from build123d import *

# Parameters (mm, degrees)
F0_R     = 11
F0_R_2   = 8.85
F0_R_3   = 8.1
F0_R_4   = 5
F1_DEPTH = 1.5
F2_DEPTH = 2.65
F3_DEPTH = 1
F4_DEPTH = 0.8


with BuildPart() as f1:
    # F0 (on Top) → F1 (new body)
    with BuildSketch(Plane.XY):
        Circle(F0_R)
        Circle(F0_R_2, mode=Mode.SUBTRACT)
        Circle(F0_R_2)
        Circle(F0_R_3, mode=Mode.SUBTRACT)
        Circle(F0_R_3)
        Circle(F0_R_4, mode=Mode.SUBTRACT)
    extrude(amount=-F1_DEPTH)

    # F0 (on Top) → F2 (join)
    with BuildSketch(Plane.XY):
        Circle(F0_R_2)
        Circle(F0_R_3, mode=Mode.SUBTRACT)
    extrude(amount=F2_DEPTH)

    # F3 (add): a face of the model
    f3_faces = [f1.faces().sort_by_distance(p)[0] for p in [
        (-8.5996841995, 0, 2.65),
    ]]
    extrude(f3_faces, amount=F3_DEPTH)

    # F4 (add): a face of the model
    f4_faces = [f1.faces().sort_by_distance(p)[0] for p in [
        (-7.8708974029, 0, 0),
    ]]
    extrude(f4_faces, amount=F4_DEPTH)


solid = f1.part
The listing builds one solid part. Answer for the finished solid, in the listing's coordinates (mm). A direction names the side the tool comes from. Round coordinates to 2 decimals unless told otherwise and drop trailing zeros. Write each loop counter-clockwise with the first axis right and the second up, starting at its lowest first coordinate (ties: lowest second). Pieces come first, ordered by that corner, then holes. Notation, with made-up numbers: (31.5, 53) - (76.5, 53) arc R32 cw to (76.5, 79) - close; hole circle Ø2 at (61.25, 68.25). An arc over 180 degrees is marked (long way). Use one line per item in the form item = value. Start each with the question number.
Item 1: A cutting plane is placed at A-A (x = 0). Write down the section's boundary in (y, z), plus the area to 3 significant figures.
Item 2: A cutting plane is placed at D-D (x = 8.5). Write down the section's boundary in (y, z).
Item 3: Determine the mould class of faces 3 (the flat face through (5.3, 0.1, 0.8)), 4 (the flat face through (2, -5, -1.5)), 5 (the cylindrical face through (-2.38, -10.74, -0.74)) for opening direction Y: +Y half, -Y half, draft (parallel to the pull), parting line (faces both ways), or undercut.
Item 4: Flat-ended cylindrical pins translate along their axes: pin 1 Ø8 at (x, y) = (-2.5, 2) entering from -Z; pin 2 Ø1 at (y, z) = (-7.5, 2.5) entering from -X (3 decimals); pin 3 Ø13 at (x, y) = (0, 0) entering from +Z. Find the tip coordinate at first contact, or state that the pin passes through.
Item 5: A cutting plane is placed at C-C (z = 1.1). Write down the section's boundary in (x, y).
Item 6: A tool of negligible diameter and unlimited length cuts with its end or side. For faces 1 (the cylindrical face through (8.44, 2.66, 1.8)), 2 (the flat face through (8, -3, 3.65)), from which of +Z, -Z, +X, -X, +Y, -Y can it reach the whole face along a straight path? Write none if from no direction.
Item 7: Find the intervals of material crossed by line 1 (Y direction, x = 0, z = 2.65); line 2 (Y direction, x = 0, z = -0.1); line 3 (Z direction, x = -3, y = 5), in increasing order. Write a range as [from, to].
The answers:
q1.outline = (-11, -1.5) - (-5, -1.5) - (-5, 0.8) - (-8.1, 0.8) - (-8.1, 3.65) - (-8.85, 3.65) - (-8.85, 0) - (-11, 0) - close; (5, -1.5) - (11, -1.5) - (11, 0) - (8.85, 0) - (8.85, 3.65) - (8.1, 3.65) - (8.1, 0.8) - (5, 0.8) - close
q1.area = 28.4 mm^2
q2.outline = (-6.98, -1.5) - (6.98, -1.5) - (6.98, 0) - (2.46, 0) - (2.46, 3.65) - (-2.46, 3.65) - (-2.46, 0) - (-6.98, 0) - close
q3.face_3 = undercut
q3.face_4 = draft
q3.face_5 = parting line
q4.pin_1 = -1.5
q4.pin_2 = -5.415
q4.pin_3 = 0.8
q5.outline = circle Ø17.7 at (0, 0); hole circle Ø16.2 at (0, 0)
q6.face_1 = +Z
q6.face_2 = +Z, +X, -X, +Y, -Y
q7.line_1 = [-8.85, -8.1], [8.1, 8.85]
q7.line_2 = [-11, -5], [5, 11]
q7.line_3 = [-1.5, 0.8]
